Answer from the drawing. Dimensions are ordinates in mm from the lowest x, y and z of the part. A direction names the side the tool comes from. Round coordinates to 2 decimals unless told otherwise and drop trailing zeros. Write each loop counter-clockwise with the first axis right and the second up, starting at its lowest first coordinate (ties: lowest second). Pieces come first, ordered by that corner, then holes. Notation, with made-up numbers: (12.5, 76) -> (47.5, 76) arc R17 ccw to (47.5, 92) -> close; hole circle Ø9 at (6, -39.75). An arc over 180 degrees is marked (long way). Return JSON: item names as keys, results as strings. Group by question number.
(1) A cutting plane is placed at B-B on y = 4.5. Give the vertices of the cut face in (x, z).
(2) A cutting plane is placed at A-A on z = 60. Give the vertices of the cut face in (x, y), then the cut area to 3 significant figures.
(3) Straight lines are drawn through the part: line 1 (X direction, y = 15.75, z = 60); line 2 (X direction, y = 12.75, z = 21.5). For each, find the intervals that lie inside material, in ascending order.
(4) The mould has two halves that part along X. Classify the marked faces 1, 2 and 3: released by +X, released by -X, zero draft, split by the parting line, or undercut.
(5) A cutting plane is placed at C-C on x = 60. Give the vertices of the cut face in (y, z).
(6) For the marked faces 4 and 5, determine the directions among +Z, -Z, +X, -X, +Y, -Y from which every point of the face is accessible in a straight line to the end or side of a thin tool.
(7) Given pin 1 (15.5 mm diameter, centred on x = 58.5, z = 17.5, fed in from -Y); pin 2 (7 mm diameter, centred on x = 40, z = 40, fed in from -Y); pin 3 (11 mm diameter, centred on x = 60, z = 60, fed in from -Y), each flat-ended and moving along its own axis, determine where each tip first touches the part or whether it passes through.
(8) A cutting plane is placed at D-D on z = 40. Give the vertices of the cut face in (x, y), then the cut area to 3 significant figures.
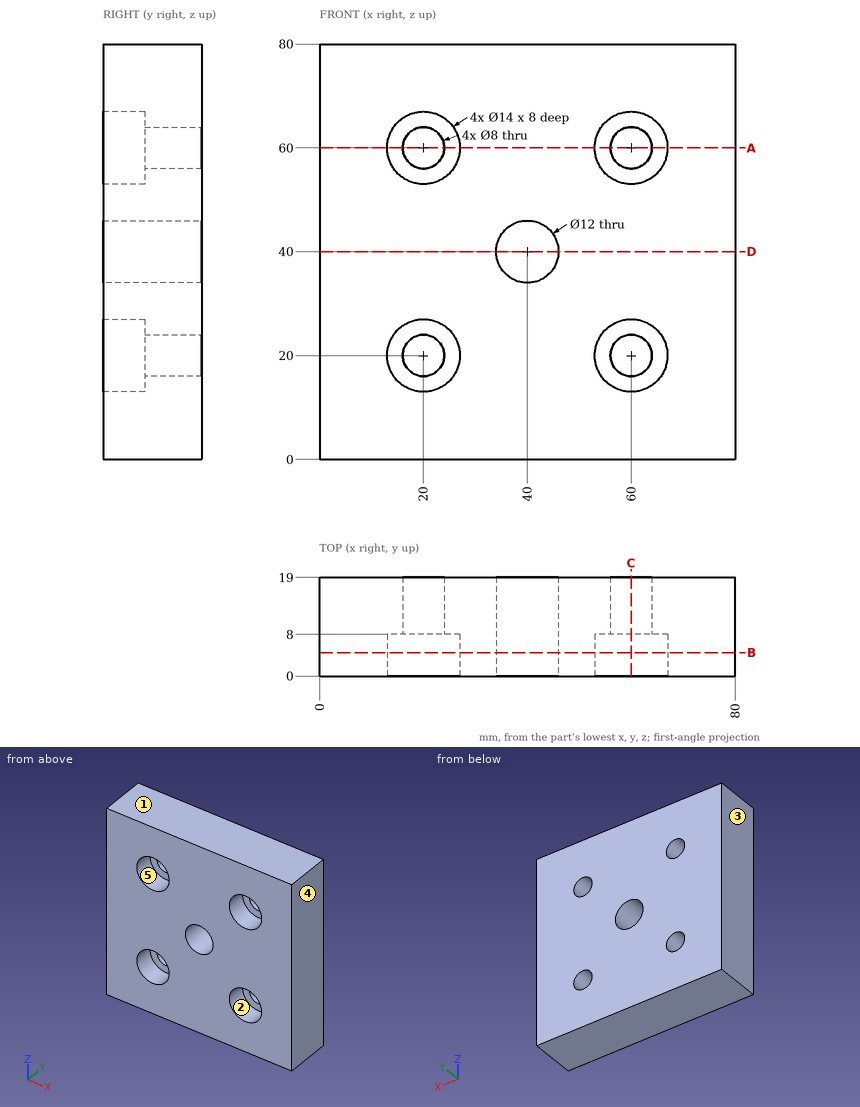
Checks:
{
 "1": {"outline": "(0, 0) -> (80, 0) -> (80, 80) -> (0, 80) -> close; hole circle Ø14 at (20, 20); hole circle Ø14 at (20, 60); hole circle Ø12 at (40, 40); hole circle Ø14 at (60, 20); hole circle Ø14 at (60, 60)"},
 "2": {"outline": "(0, 0) -> (13, 0) -> (13, 8) -> (16, 8) -> (16, 19) -> (0, 19) -> close; (24, 8) -> (27, 8) -> (27, 0) -> (53, 0) -> (53, 8) -> (56, 8) -> (56, 19) -> (24, 19) -> close; (64, 8) -> (67, 8) -> (67, 0) -> (80, 0) -> (80, 19) -> (64, 19) -> close", "area": "1,120 mm^2"},
 "3": {"line 1": "x = 0 to 16, 24 to 56, 64 to 80", "line 2": "x = 0 to 16.29, 23.71 to 56.29, 63.71 to 80"},
 "4": {"face 1": "zero draft", "face 2": "undercut", "face 3": "released by -X"},
 "5": {"outline": "(0, 0) -> (19, 0) -> (19, 16) -> (8, 16) -> (8, 13) -> (0, 13) -> close; (0, 27) -> (8, 27) -> (8, 24) -> (19, 24) -> (19, 56) -> (8, 56) -> (8, 53) -> (0, 53) -> close; (0, 67) -> (8, 67) -> (8, 64) -> (19, 64) -> (19, 80) -> (0, 80) -> close"},
 "6": {"face 4": "+Z, -Z, +X, +Y, -Y", "face 5": "-Y"},
 "7": {"pin 1": "stops at y = 0", "pin 2": "passes through", "pin 3": "stops at y = 8"},
 "8": {"outline": "(0, 0) -> (34, 0) -> (34, 19) -> (0, 19) -> close; (46, 0) -> (80, 0) -> (80, 19) -> (46, 19) -> close", "area": "1,290 mm^2"}
}
